from build123d import *

# Parameters (mm, degrees)
BOSS_EXTRUDE1_DEPTH = 15
SKETCH2_R           = 0.85
CUT_EXTRUDE1_DEPTH  = 20


with BuildPart() as part:
    # Sketch1 → Boss-Extrude1 (new body, symmetric)
    with BuildSketch(Plane(origin=(0, 0, 0), x_dir=(1, 0, 0), z_dir=(0, 1, 0))):
        Polygon((-3, 10), (-3, -3), (10, -3), (10, -9), (-9, -9), (-9, 10), align=None)
    extrude(amount=BOSS_EXTRUDE1_DEPTH, both=True)

    # Sketch2 → Cut-Extrude1 (cut, through all)
    with BuildSketch(Plane.XY.offset(9)):
        with Locations((6.35, 6.35)):
            Circle(SKETCH2_R)
        with Locations((6.35, 0)):
            Circle(SKETCH2_R)
        with Locations((6.35, -6.35)):
            Circle(SKETCH2_R)
    cut_extrude1 = extrude(amount=-CUT_EXTRUDE1_DEPTH, mode=Mode.SUBTRACT)

    # Mirror1: Cut-Extrude1 across plane
    add(cut_extrude1.mirror(Plane(origin=(0, 0, 0), x_dir=(-0.707106781, 0, 0.707106781), z_dir=(0.707106781, 0, 0.707106781))), mode=Mode.SUBTRACT)


solid = part.part
Design review of the part built by this model. Coordinates are the model's own, in mm. A direction names the side the tool comes from. Coordinates: 2 decimals unless noted, no trailing zeros. Loops run counter-clockwise (first coordinate to the right, second up) from the corner with the lowest first, then second, coordinate; pieces in that order, holes last. Notation, with made-up numbers: (-26, -39.75) -> (-13, -39.75) arc R31 ccw to (-13, -4.75) -> close; hole circle Ø7 at (42, 20.5). An arc over 180 degrees is marked (long way). Use a Markdown table: item, result. Add a question column.
Item 1: Wall thickness on L1, parallel to Y at x = 6.35, z = 6; L2, parallel to Z at x = -2, y = 8; L3, parallel to Z at x = -5.75, y = 6.5: over which ranges is each line inside the solid? List them lowest first. Write a range as from..to.
Item 2: We need section D-D, the plane y = 1.5. Write out the cut boundary in (x, z).
Item 3: Clearance check with flat-ended pins moving along their axes: P1, Ø2, axis at x = 6.35, y = -6.35, coming from the -Z side; P2, Ø2, axis at y = 6.35, z = -6.35, coming from the +X side; P3, Ø1, axis at y = -6.35, z = -6.35, coming from the -X side. State where each tip first meets the part, or that it passes through.
Item 4: We need section B-B, the plane z = -6.35. Write out the cut boundary in (x, y), and give its area (3 significant figures).
Item 5: Machinability: for faces 1 (the flat face through (-3, 0, -4)), 2 (the cylindrical face through (5.7, 5.8, 6)), which of the approach directions +Z, -Z, +X, -X, +Y, -Y give a long, thin tool a straight path to every point of the face, cutting with its end or side? Answer none if there is none.
Item 6: We need section A-A, the plane y = -6.35. Write out the cut boundary in (x, z), and give its area (3 significant figures).
Item 7: We need section C-C, the plane x = 6.35. Write out the cut boundary in (y, z), and give its area (3 significant figures).
Item 8: The part is to be moulded in two halves that separate along Y. For faces 3 (the cylindrical face through (5.5, -6.3, 6)), 4 (the flat face through (3, 0, 3)), 5 (the flat face through (-4, -15, 1)), say which applies: +Y half, -Y half, draft (parallel to the pull), parting line (faces both ways), or undercut.
Numbers:
| question | item | result |
|---|---|---|
| 1 | L1 | y = -15..-7.2, -5.5..-0.85, 0.85..5.5, 7.2..15 |
| 1 | L2 | z = 3..9 |
| 1 | L3 | z = -10..-7.19, -5.51..9 |
| 2 | outline | (-9, -10) -> (-3, -10) -> (-3, 3) -> (10, 3) -> (10, 9) -> (-9, 9) -> close |
| 3 | P1 | stops at z = 3 |
| 3 | P2 | stops at x = -3 |
| 3 | P3 | passes through |
| 4 | outline | (-9, -15) -> (-3, -15) -> (-3, -7.2) -> (-9, -7.2) -> close; (-9, -5.5) -> (-3, -5.5) -> (-3, -0.85) -> (-9, -0.85) -> close; (-9, 0.85) -> (-3, 0.85) -> (-3, 5.5) -> (-9, 5.5) -> close; (-9, 7.2) -> (-3, 7.2) -> (-3, 15) -> (-9, 15) -> close |
| 4 | area | 149 mm^2 |
| 5 | face 1 | -Z, +X, +Y, -Y |
| 5 | face 2 | +Z, -Z |
| 6 | outline | (-9, -10) -> (-3, -10) -> (-3, -7.2) -> (-9, -7.2) -> close; (-9, -5.5) -> (-3, -5.5) -> (-3, 3) -> (5.5, 3) -> (5.5, 9) -> (-9, 9) -> close; (7.2, 3) -> (10, 3) -> (10, 9) -> (7.2, 9) -> close |
| 6 | area | 172 mm^2 |
| 7 | outline | (-15, 3) -> (-7.2, 3) -> (-7.2, 9) -> (-15, 9) -> close; (-5.5, 3) -> (-0.85, 3) -> (-0.85, 9) -> (-5.5, 9) -> close; (0.85, 3) -> (5.5, 3) -> (5.5, 9) -> (0.85, 9) -> close; (7.2, 3) -> (15, 3) -> (15, 9) -> (7.2, 9) -> close |
| 7 | area | 149 mm^2 |
| 8 | face 3 | undercut |
| 8 | face 4 | draft |
| 8 | face 5 | -Y half |
